Autodesk Inventor part; units mm, degrees
ref_plane "YZ Plane" through (0, 0, 0) normal (1, 0, 0) x (0, 1, 0)
ref_plane "XZ Plane" through (0, 0, 0) normal (0, 1, 0) x (-1, 0, 0)
ref_plane "XY Plane" through (0, 0, 0) normal (0, 0, 1) x (1, 0, 0)
sketch "Sketch1" plane through (0, 0, 0) normal (0, 1, 0) x (-1, 0, 0)
  point P0 (0, 0)
sketch "Sketch2" plane through (-2.6971, 0, -13.0721) normal (0, 1, 0) x (-1, 0, 0)
  circle A0 centre (-1.6971, 1.6971) radius 2.5
  line L0 (2.3029, 5.6971) -> (-5.6971, 5.6971)
  line L1 (-5.6971, 5.6971) -> (-5.6971, -2.3029)
  line L2 (-5.6971, -2.3029) -> (2.3029, -2.3029)
  line L3 (2.3029, -2.3029) -> (2.3029, 5.6971)
  line L4 (2.3029, 5.6971) -> (-5.6971, -2.3029) construction
  line L5 (-5.6971, 5.6971) -> (2.3029, -2.3029) construction
  line L6 (2.3029, 5.6971) -> (-5.6971, 5.6971)
  line L7 (-5.6971, 5.6971) -> (-5.6971, 35.6971)
  line L8 (-5.6971, 35.6971) -> (2.3029, 35.6971)
  line L9 (2.3029, 35.6971) -> (2.3029, 5.6971)
  point P0 (-7.6971, -4.5529)
  dimension "d3" = 5
  dimension "d1" = 8
  dimension "d2" = 8
  dimension "d0" = 30
extrude "Extrusion1" add sketch "Sketch2" along normal blind 5
sketch "Sketch3" plane through (-2.6971, 0, -13.0721) normal (0, -1, 0) x (1, 0, 0)
  line L0 (-2.3029, -2.3029) -> (-2.3029, 35.6971)
  line L1 (5.6449, 20.1971) -> (-2.3029, 20.1971)
  line L2 (-2.3029, 20.1971) -> (-2.3029, 17.1971)
  line L3 (-2.3029, 17.1971) -> (5.6449, 17.1971)
  line L4 (5.6449, 17.1971) -> (5.6449, 20.1971)
  line L5 (5.6449, 32.6971) -> (-2.3029, 32.6971)
  line L6 (-2.3029, 32.6971) -> (-2.3029, 35.6971)
  line L7 (-2.3029, 35.6971) -> (5.6449, 35.6971)
  line L8 (5.6449, 35.6971) -> (5.6449, 32.6971)
  point P0 (2.6971, 13.0721)
  dimension "d7" = 3
  dimension "d11" = 12.5
  dimension "d12" = 3
extrude "Extrusion2" add sketch "Sketch3" along normal blind 23
sketch "Sketch4" plane through (-5, 0, -15.375) normal (-1, 0, 0) x (0, 0, 1)
  point P0 (15.375, 0)
properties part number "A1"
Read the model definition and answer for the solid it produces. Units are mm, in the model's axes. A direction names the side the tool comes from. Coordinates: 2 decimals unless noted, no trailing zeros. Write each loop counter-clockwise with the first axis right and the second up, starting at its lowest first coordinate (ties: lowest second). Pieces come first, ordered by that corner, then holes. Notation, with made-up numbers: (42, -16) -> (49, -16) arc R15 cw to (49, 8) -> close; hole circle Ø11 at (87.5, 22). An arc over 180 degrees is marked (long way). Return JSON: item names as keys, results as strings.
1. A tool of negligible diameter and unlimited length cuts with its end or side. For faces 1 (the face through (2.948, -11, 6)), 2 (the face through (-1, -11, 19.625)), 3 (the face through (-1, -23, 6)), from which of +Z, -Z, +X, -X, +Y, -Y can it reach the whole face along a straight path? Write none if from no direction.
Found:
{"face 1": "+Z, -Z, +X, -Y", "face 2": "+X, -X, -Y", "face 3": "+Z, -Z, +X, -X, -Y"}
2. Find the intervals of material crossed by line 1 along Z through (x, y) = (-1, 1.2) (3 decimals); line 2 along Z through (x, y) = (-0.25, -8.25) (3 decimals); line 3 along Y through (x, z) = (-0.5, 1.5), in increasing order. Write a range as from..to.
Found:
{"line 1": "-15.375..-13.875, -8.875..22.625", "line 2": "4.125..7.125, 19.625..22.625", "line 3": "0..5"}
3. Each of these flat-tipped pins is pushed along its axis until it touches: P1, Ø8, axis at y = -4.5, z = 4.5, coming from the +X side; P2, Ø1.5, axis at x = 0.5, z = 17, coming from the -Y side; P3, Ø2.5, axis at x = -1, y = -13.5, coming from the -Z side (3 decimals). Where does it stop, or does it pass through?
Found:
{"P1": "x = 2.95", "P2": "y = 0", "P3": "z = 4.125"}
4. A cutting plane is placed at A-A (x = -1). Determine the outline of the cut face in (y, z) (3 decimals), and give its area (3 significant figures).
Found:
{"outline": "(-23, 4.125) -> (0, 4.125) -> (0, -8.875) -> (5, -8.875) -> (5, 22.625) -> (-23, 22.625) -> (-23, 19.625) -> (0, 19.625) -> (0, 7.125) -> (-23, 7.125) -> close; (0, -15.375) -> (5, -15.375) -> (5, -13.875) -> (0, -13.875) -> close", "area": "303 mm2"}
5. Determine the mould class of faces 4 (the face through (-1, -11, 4.125)), 5 (the face through (-1, -11, 7.125)), 6 (the face through (-1, -9, 22.625)), 7 (the face through (-0.458, 2.465, -8.934)) for opening direction Z: pulls with the +Z half, pulls with the -Z half, needs draft (parallel to the pull), parting line crosses it, or undercut.
Found:
{"face 4": "pulls with the -Z half", "face 5": "undercut", "face 6": "pulls with the +Z half", "face 7": "undercut"}
6. A cutting plane is placed at B-B (y = -7.75). Determine the outline of the cut face in (x, z) (3 decimals).
Found:
{"outline": "(-5, 4.125) -> (2.948, 4.125) -> (2.948, 7.125) -> (-5, 7.125) -> close; (-5, 19.625) -> (2.948, 19.625) -> (2.948, 22.625) -> (-5, 22.625) -> close"}
7. A cutting plane is placed at C-C (z = 2). Determine the outline of the cut face in (x, y), and give its area (3 significant figures).
Found:
{"outline": "(-5, 0) -> (3, 0) -> (3, 5) -> (-5, 5) -> close", "area": "40.0 mm2"}
